For this review, take the finished solid that the model builds, in its own axes (mm). A direction names the side the tool comes from. Give positions to 0.01 mm unless a question says otherwise; leave off trailing zeros. Write each loop counter-clockwise with the first axis right and the second up, starting at its lowest first coordinate (ties: lowest second). Pieces come first, ordered by that corner, then holes. Notation, with made-up numbers: M 47.5,15 L 86.5,15 A21 cw 86.5,33 Z; hole C 11.5,-2 d6. An arc over 180 degrees is marked long. Use one line per item in the form item = value. Start each with the question number.
Q1. For probe 1 along Y at (x, z) = (3.25, 0); probe 2 along Y at (x, z) = (3, 11.5); probe 3 along Z at (x, y) = (5, -7.85), list the stretches that pass through material, from the lowest coordinate up. Write a range as [from, to].
Q2. Clearance check with flat-ended pins moving along their axes: pin 1 Ø2.5 at (x, z) = (5, 12.5) entering from -Y; pin 2 Ø4 at (x, y) = (8, 2) entering from +Z; pin 3 Ø4 at (x, z) = (5, 9) entering from +Y; pin 4 Ø1 at (x, y) = (5, 5.5) entering from -Z. State where each tip first meets the part, or that it passes through.
Q3. Consider section A-A on x = 5. Write out the cut boundary in (y, z).
Q4. Consider section B-B on z = -20.5. Write out the cut boundary in (x, y).
Q5. Consider section D-D on z = 0. Write out the cut boundary in (x, y).
Q6. Tool access review of faces 1 (the flat face through (0, -3, -4)), 2 (the flat face through (5, 2, -16.5)): name each direction out of +Z, -Z, +X, -X, +Y, -Y from which nothing blocks a thin tool from reaching the whole face with its end or side.
Q7. Mouldability with a two-part tool opening along Y and no side actions: class faces 3 (the flat face through (6, -6.25, 11)), 4 (the cylindrical face through (4.93, 9.804, -0.672)), 5 (the flat face through (5, -10, -24.5)) as released by +Y, released by -Y, zero draft, split by the parting line, or undercut.
Q8. Consider section C-C on y = -8.75. Write out the cut boundary in (x, z).
```python
from build123d import *

# Parameters (mm, degrees)
SKETCH1_W           = 25
SKETCH1_H           = 22.5
SKETCH1_R           = 1.25
BOSS_EXTRUDE1_DEPTH = 10
SKETCH4_W           = 10
SKETCH4_H           = 5
BOSS_EXTRUDE3_DEPTH = 8
SKETCH5_W           = 10
SKETCH5_H           = 5
BOSS_EXTRUDE4_DEPTH = 8
FILLET1_R           = 2
CUT_EXTRUDE1_REACH  = 7
SKETCH6_R           = 1.55
CUT_EXTRUDE2_REACH  = 7
SKETCH7_R           = 1.55


with BuildPart() as part:
    # Sketch1 → Boss-Extrude1 (new body)
    with BuildSketch(Plane(origin=(0, 0, 0), x_dir=(0, 0, -1), z_dir=(1, 0, 0))):
        with Locations((4, 0)):
            Rectangle(SKETCH1_W, SKETCH1_H)
        with Locations((0, 8.75)):
            Circle(SKETCH1_R, mode=Mode.SUBTRACT)
        with Locations((0, -8.75)):
            Circle(SKETCH1_R, mode=Mode.SUBTRACT)
    extrude(amount=BOSS_EXTRUDE1_DEPTH)

    # Sketch4 → Boss-Extrude3 (add)
    with BuildSketch(Plane(origin=(0, 0, -16.5), x_dir=(-1, 0, 0), z_dir=(0, 0, -1))):
        with Locations((-5, -8.75)):
            Rectangle(SKETCH4_W, SKETCH4_H)
    extrude(amount=BOSS_EXTRUDE3_DEPTH)

    # Sketch5 → Boss-Extrude4 (add)
    with BuildSketch(Plane.XY.offset(8.5)):
        with Locations((5, -8.75)):
            Rectangle(SKETCH5_W, SKETCH5_H)
    extrude(amount=BOSS_EXTRUDE4_DEPTH)

    # Fillet1
    fillet1_edges = [part.edges().sort_by_distance(p)[0] for p in [
        (5, -6.25, 8.5),
        (5, -6.25, 16.5),
        (5, -6.25, -24.5),
        (5, -6.25, -16.5),
        (5, 11.25, -16.5),
        (5, 11.25, 8.5),
    ]]
    fillet(fillet1_edges, radius=FILLET1_R)

    # Sketch6 → Cut-Extrude1 (cut, up to next)
    with BuildSketch(Plane(origin=(0, -6.25, 0), x_dir=(1, 0, 0), z_dir=(0, 1, 0)), mode=Mode.PRIVATE) as cut_extrude1_sk1:
        with Locations((5, -12.5)):
            Circle(SKETCH6_R)
    cut_extrude1_tool1 = extrude(cut_extrude1_sk1.sketch, amount=-CUT_EXTRUDE1_REACH, mode=Mode.PRIVATE) & part.part
    add(cut_extrude1_tool1.solids().sort_by_distance((5, -6.25, 12.5))[0], mode=Mode.SUBTRACT)

    # Sketch7 → Cut-Extrude2 (cut, up to next)
    with BuildSketch(Plane(origin=(0, -6.25, 0), x_dir=(1, 0, 0), z_dir=(0, 1, 0)), mode=Mode.PRIVATE) as cut_extrude2_sk1:
        with Locations((5, 20.5)):
            Circle(SKETCH7_R)
    cut_extrude2_tool1 = extrude(cut_extrude2_sk1.sketch, amount=-CUT_EXTRUDE2_REACH, mode=Mode.PRIVATE) & part.part
    add(cut_extrude2_tool1.solids().sort_by_distance((5, -6.25, -20.5))[0], mode=Mode.SUBTRACT)


solid = part.part
```
Working result:
q1.probe_1 = [-11.25, -10], [-7.5, 7.5], [10, 11.25]
q1.probe_2 = [-11.25, -6.25]
q1.probe_3 = [-24.46, -22.05], [-18.95, -0.87], [0.87, 10.95], [14.05, 16.46]
q2.pin_1 = through
q2.pin_2 = 8.5
q2.pin_3 = 11.19
q2.pin_4 = -16.5
q3.outline = M -11.25,-24.5 L -8.25,-24.5 A2 ccw -6.25,-22.5 L -6.25,-22.05 L -11.25,-22.05 Z; M -11.25,-18.95 L -6.25,-18.95 L -6.25,-18.5 A2 cw -4.25,-16.5 L 9.25,-16.5 A2 ccw 11.25,-14.5 L 11.25,6.5 A2 ccw 9.25,8.5 L -4.25,8.5 A2 cw -6.25,10.5 L -6.25,10.95 L -11.25,10.95 Z; M -11.25,14.05 L -6.25,14.05 L -6.25,14.5 A2 ccw -8.25,16.5 L -11.25,16.5 Z; hole C -8.75,0 d2.5; hole C 8.75,0 d2.5
q4.outline = M 0,-11.25 L 3.45,-11.25 L 3.45,-6.25 L 0,-6.25 Z; M 6.55,-11.25 L 10,-11.25 L 10,-6.25 L 6.55,-6.25 Z
q5.outline = M 0,-11.25 L 10,-11.25 L 10,-10 L 0,-10 Z; M 0,-7.5 L 10,-7.5 L 10,7.5 L 0,7.5 Z; M 0,10 L 10,10 L 10,11.25 L 0,11.25 Z
q6.face_1 = +Z, -Z, -X, +Y, -Y
q6.face_2 = -Z, +X, -X, +Y
q7.face_3 = released by +Y
q7.face_4 = undercut
q7.face_5 = zero draft
q8.outline = M 0,-24.5 L 10,-24.5 L 10,-1.25 L 0,-1.25 Z; M 0,1.25 L 10,1.25 L 10,16.5 L 0,16.5 Z; hole C 5,-20.5 d3.1; hole C 5,12.5 d3.1
